Geometry: final body of the model. Coordinates: model frame, mm. Face numbers are marked on the shaded views. Give positions to 0.01 mm unless a question says otherwise; leave off trailing zeros. Write each loop counter-clockwise with the first axis right and the second up, starting at its lowest first coordinate (ties: lowest second). Pieces come first, ordered by that corner, then holes. Notation, with made-up numbers: (-35.5, -14.5) - (-17.5, -14.5) arc R16 ccw to (-17.5, -0.5) - close; hole circle Ø3 at (-37.5, 64.5). An arc over 180 degrees is marked (long way). Use CSV: the item, a comma, the result in double quotes. Start each with the question number.
(1) Draft query along Y for the marked faces 1, 2 and 3. Return one class per face: released by +Y, released by -Y, zero draft, split by the parting line, or undercut.
(2) Line query: probe 1 along Y at (x, z) = (-20, -22.5); probe 2 along Y at (x, z) = (-26, 1.5); probe 3 along Z at (x, y) = (-17.5, -36.5). Output: solid intervals per line, ascending. Write a range as [from, to].
(3) First-contact query: pin 1 Ø1 at (x, z) = (-1.5, 47.5) entering from +Y; pin 2 Ø8 at (y, z) = (-20.5, 27) entering from +X; pin 3 Ø1 at (x, z) = (-0.5, 48.5) entering from +Y. Flat tips, straight axial feed; report the tip coordinate or a pass-through.
(4) Section A-A on z = -44. Output: boundary loops of the cut face in (x, y), and give its area (3 significant figures).
(5) Section B-B on x = -8. Count the separate pieces of the cut face and the enclosed holes in it, and give its area (3 significant figures).
from build123d import *

# Parameters (mm, degrees)
F1_ANGLE_BACK = 90
F1_ANGLE      = 180
F3_DEPTH      = 49
F4_DEPTH      = 42
F5_DEPTH      = 53
F6_R          = 1.75
F7_DEPTH      = 62.5


with BuildPart() as f1:
    # F0 (on Front) → F1 (revolve)
    with BuildSketch(Plane.XZ, mode=Mode.PRIVATE) as f1_sk:
        with BuildLine():
            ThreePointArc((-35.5, 47), (-36.3786796564, 49.1213203436), (-38.5, 50))
            Line((-38.5, 50), (-49, 50))
            add(Edge.make_bspline(
                [(-49, 50), (-50.0905438599, 49.4592544488), (-53.0493875637, 47.4989733534), (-57.4486951492, 41.931344871), (-61.5763053799, 28.0443008729), (-61.4881986154, 14.5014666819), (-62, 0)],
                knots=[0, 0, 0, 0, 0.1531073754, 0.3436852098, 0.6019385566, 1, 1, 1, 1], degree=3))
            Line((-62, 0), (-62, -50))
            Line((-62, -50), (-59.5, -50))
            Line((-59.5, -50), (-59.5, 0))
            add(Edge.make_bspline(
                [(-51.1955396277, 43), (-59.7999691963, 32.3488041759), (-58.4857873619, 15.5563373119), (-59.5, 0)],
                knots=[0, 0, 0, 0, 43.7945665817, 43.7945665817, 43.7945665817, 43.7945665817], degree=3))
            Line((-51.1955396277, 43), (-38.5, 43))
            ThreePointArc((-38.5, 43), (-36.3786796564, 43.8786796564), (-35.5, 46))
            Line((-35.5, 46), (-35.5, 47))
        make_face()
    revolve(f1_sk.sketch.rotate(Axis((0, 0, -47.5967168808), (0, 0, 1)), -F1_ANGLE_BACK), axis=Axis((0, 0, -47.5967168808), (0, 0, 1)), revolution_arc=F1_ANGLE)

    # F2 (on Front) → F3 (cut)
    with BuildSketch(Plane.XZ):
        with BuildLine():
            ThreePointArc((0, 45), (1.4142135624, 45.5857864376), (2, 47))
            ThreePointArc((2, 47), (1.4142135624, 48.4142135624), (0, 49))
            ThreePointArc((0, 49), (-1.3909130574, 48.4371363424), (-1.998931704, 47.0653608667))
            Line((-1.998931704, 47.0653608667), (-1.998931704, 46.9346391333))
            ThreePointArc((-1.998931704, 46.9346391333), (-1.3909130574, 45.5628636576), (0, 45))
        make_face()
    extrude(amount=F3_DEPTH, mode=Mode.SUBTRACT)

    # F2 (on Front) → F4 (cut)
    with BuildSketch(Plane.XZ):
        with BuildLine():
            ThreePointArc((-1.998931704, 47.0653608667), (-1.3909130574, 48.4371363424), (0, 49))
            Line((0, 49), (0, 50.3604523001))
            Line((0, 50.3604523001), (-1.998931704, 50.3604523001))
            Line((-1.998931704, 50.3604523001), (-1.998931704, 47.0653608667))
        make_face()
    extrude(amount=F4_DEPTH, mode=Mode.SUBTRACT)

    # F2 (on Front) → F5 (cut)
    with BuildSketch(Plane.XZ):
        with BuildLine():
            Line((0, 41.0653608667), (0, 45))
            ThreePointArc((0, 45), (-1.3909130574, 45.5628636576), (-1.998931704, 46.9346391333))
            Line((-1.998931704, 46.9346391333), (-1.998931704, 41.0653608667))
            Line((-1.998931704, 41.0653608667), (0, 41.0653608667))
        make_face()
    extrude(amount=F5_DEPTH, mode=Mode.SUBTRACT)

    # F6 (on Front) → F7 (cut, symmetric)
    with BuildSketch(Plane.XZ):
        with Locations((-8, -44)):
            Circle(F6_R)
    extrude(amount=F7_DEPTH, both=True, mode=Mode.SUBTRACT)


solid = f1.part
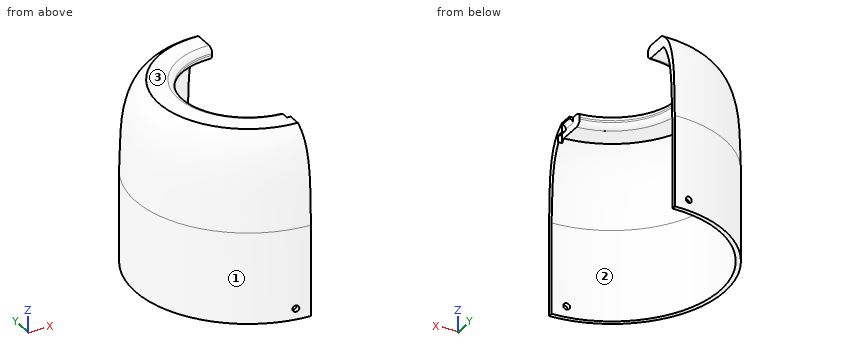
Check values:
1,face 1,"split by the parting line"
1,face 2,"undercut"
1,face 3,"zero draft"
2,probe 1,"y = [-58.69, -56.04], [56.04, 58.69]"
2,probe 2,"y = [-56.23, -53.42], [53.42, 56.23]"
2,probe 3,"z = [43, 50]"
3,pin 1,"stops at y = 53.12"
3,pin 2,"stops at x = -52.04"
3,pin 3,"stops at y = 52.02"
4,outline,"(-9.75, -61.23) - (-9.75, -58.7) arc R59.5 cw to (-9.75, 58.7) - (-9.75, 61.23) arc R62 ccw to start; (-6.25, -61.68) arc R62 ccw to (0, -62) - (0, -59.5) arc R59.5 cw to (-6.25, -59.17) - close; (-6.25, 59.17) arc R59.5 cw to (0, 59.5) - (0, 62) arc R62 ccw to (-6.25, 61.68) - close"
4,area,"459 mm²"
5,separate pieces,"4"
5,enclosed holes,"0"
5,area,"752 mm²"
